Autodesk Inventor part; units mm, degrees
ref_plane "Work Plane1" through (0, 5, 0) normal (0, 1, 0) x (1, 0, 0)
ref_plane "Work Plane2" through (0, 80, 0) normal (0, 1, 0) x (1, 0, 0)
ref_plane "Work Plane3" through (-25, 0, 27) normal (0, 0, 1) x (1, 0, 0)
sketch "Sketch1" plane through (0, 0, 0) normal (0, 1, 0) x (-1, 0, 0)
  line L0 (27, 27) -> (-27, 27)
  line L1 (-27, 27) -> (-27, -27)
  line L2 (-27, -27) -> (27, -27)
  line L3 (27, -27) -> (27, 27)
  line L4 (27, 27) -> (-27, -27) construction
  line L5 (-27, 27) -> (27, -27) construction
  circle A0 centre (25, 25) radius 1
  circle A1 centre (25, -25) radius 1
  circle A2 centre (-25, -25) radius 1
  circle A3 centre (-25, 25) radius 1
  point P0 (0, 0)
  dimension "d0" = 54
  dimension "d1" = 54
  dimension "d2" = 2
  dimension "d3" = 2
  dimension "d4" = 2
  dimension "d5" = 2
extrude "Extrusion1" add sketch "Sketch1" along normal blind 5
fillet "Fillet1" radius 2 1 edges at (27, 2.5, -27)
fillet "Fillet2" radius 2 3 edges at (-27, 2.5, -27) (-27, 2.5, 27) (27, 2.5, 27)
ref_plane "Work Plane1" through (0, 5, 0) normal (0, 1, 0) x (1, 0, 0)
sketch "Sketch3" plane through (0, 5, 0) normal (0, 1, 0) x (1, 0, 0)
  circle A0 centre (0, 0) radius 25
  line L0 (-25, -27) -> (25, -27)
  line L1 (0, -27) -> (20, -27)
  line L2 (20, -27) -> (20, -15)
  line L3 (0, -27) -> (-20, -27)
  line L4 (-20, -27) -> (-20, -15)
  dimension "d11" = 50
  dimension "d12" = 20
  dimension "d13" = 20
extrude "Extrusion2" add sketch "Sketch3" along normal blind 75
ref_plane "Work Plane2" through (0, 80, 0) normal (0, 1, 0) x (1, 0, 0)
sketch "Sketch4" plane through (0, 80, 0) normal (0, 1, 0) x (1, 0, 0)
  circle A0 centre (0, 0) radius 20
  dimension "d17" = 40
extrude "Extrusion3" cut sketch "Sketch4" against normal blind 5
ref_plane "Work Plane3" through (-25, 0, 27) normal (0, 0, 1) x (1, 0, 0)
sketch "Sketch5" plane through (-25, 0, 27) normal (0, 0, 1) x (1, 0, 0)
  line L0 (25, 0) -> (25, 7.5)
  line L1 (5, 15) -> (45, 15)
  line L2 (45, 15) -> (45, 0)
  line L3 (45, 0) -> (5, 0)
  line L4 (5, 0) -> (5, 15)
  line L5 (5, 15) -> (45, 0) construction
  line L6 (45, 15) -> (5, 0) construction
  dimension "d21" = 7.5
  dimension "d22" = 40
  dimension "d23" = 15
extrude "Extrusion4" add sketch "Sketch5" along normal blind 5
ref_plane "Work Plane4" through (-25, 0, 32) normal (0, 0, 1) x (1, 0, 0)
sketch "Sketch6" plane through (-25, 0, 32) normal (0, 0, 1) x (1, 0, 0)
  line L0 (25, 7.5) -> (25, 8.92)
  circle A0 centre (25, 8.92) radius 0.5
  line L1 (25, 8.92) -> (27.3, 8.92)
  line L2 (27.3, 8.92) -> (29.6, 8.92)
  line L3 (25, 8.92) -> (22.7, 8.92)
  line L4 (22.7, 8.92) -> (20.4, 8.92)
  circle A1 centre (20.4, 8.92) radius 0.5
  circle A2 centre (27.3, 8.92) radius 0.5
  circle A3 centre (22.7, 8.92) radius 0.5
  circle A4 centre (29.6, 8.92) radius 0.5
  line L5 (25, 7.5) -> (25, 6.08)
  line L6 (26.15, 6.08) -> (25, 6.08)
  line L7 (23.85, 6.08) -> (25, 6.08)
  circle A5 centre (26.15, 6.08) radius 0.5
  circle A6 centre (23.85, 6.08) radius 0.5
  line L8 (23.85, 6.08) -> (21.55, 6.08)
  line L9 (26.15, 6.08) -> (28.45, 6.08)
  circle A7 centre (28.45, 6.08) radius 0.5
  circle A8 centre (21.55, 6.08) radius 0.5
  line L10 (18.3522, 10.2186) -> (31.6478, 10.2186)
  line L11 (30.8187, 4.7814) -> (19.1813, 4.7814)
  line L12 (31.6478, 10.2186) -> (30.8187, 4.7814)
  line L13 (18.3522, 10.2186) -> (19.1813, 4.7814)
  line L14 (25, 10.2186) -> (25, 11.0186)
  line L15 (25, 4.7814) -> (25, 3.9814)
  line L16 (25, 3.9814) -> (31.5285, 3.9814)
  line L17 (31.5285, 3.9814) -> (32.5973, 11.0186)
  line L18 (32.5973, 11.0186) -> (25, 11.0186)
  line L19 (25, 3.9814) -> (18.4715, 3.9814)
  line L20 (18.4715, 3.9814) -> (17.4027, 11.0186)
  line L21 (17.4027, 11.0186) -> (25, 11.0186)
  point P0 (25, 0)
  dimension "d30" = 1
  dimension "d33" = 1
  dimension "d34" = 1
  dimension "d35" = 1
  dimension "d36" = 1
  dimension "d38" = 1
  dimension "d39" = 1
  dimension "d40" = 1
  dimension "d41" = 1
  dimension "d44" = 0.8
extrude "Extrusion5" add sketch "Sketch6" along normal blind 10 contours A1 | A3 L4 L3 | L3 L4 A3 | A4 | A2 L2 L1 | L1 L2 A2 | A0 L3 L0 | L0 L1 A0 | A7 | A5 L9 L6 | L6 L9 A5 | A8 | A6 L8 L7 | L7 L8 A6 | L3 A0 L1 | L13 L11 L15 L19 L20 L21 L14 L10 | L14 L18 L17 L16 L15 L11 L12 L10
sketch "Sketch7" plane through (-25, 0, 32) normal (0, 0, 1) x (1, 0, 0)
  line L0 (5, 15) -> (5, 0)
  line L1 (5, 7.5) -> (10, 7.5)
  circle A0 centre (10, 7.5) radius 1.5
  line L2 (12.3579, 7.5) -> (11.1789, 5.458)
  line L3 (11.1789, 5.458) -> (8.8211, 5.458)
  line L4 (8.8211, 5.458) -> (7.6421, 7.5)
  line L5 (7.6421, 7.5) -> (8.8211, 9.542)
  line L6 (8.8211, 9.542) -> (11.1789, 9.542)
  line L7 (11.1789, 9.542) -> (12.3579, 7.5)
  line L8 (25, 0) -> (25, 2.1902)
  circle A1 centre (40, 7.5) radius 1.5
  line L9 (37.6421, 7.5) -> (38.8211, 5.458)
  line L10 (38.8211, 5.458) -> (41.1789, 5.458)
  line L11 (41.1789, 5.458) -> (42.3579, 7.5)
  line L12 (42.3579, 7.5) -> (41.1789, 9.542)
  line L13 (41.1789, 9.542) -> (38.8211, 9.542)
  line L14 (38.8211, 9.542) -> (37.6421, 7.5)
  dimension "d48" = 5
  dimension "d49" = 3
extrude "Extrusion6" add sketch "Sketch7" along normal blind 10
properties part number "sensor 1"
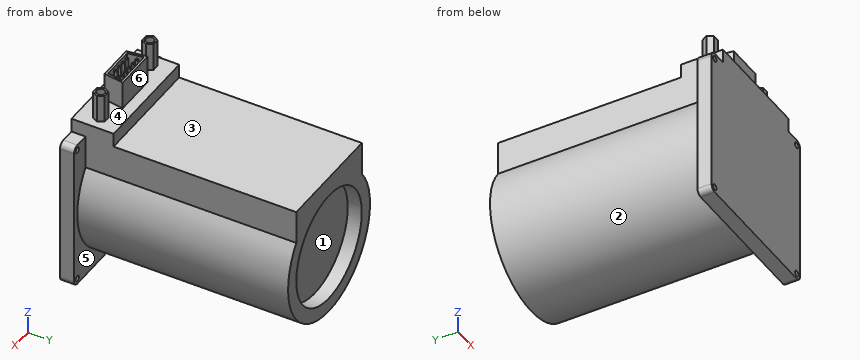
Read the model definition and answer for the solid it produces. Units are mm, in the model's axes. Face numbers are marked on the shaded views. A direction names the side the tool comes from. Round coordinates to 2 decimals unless told otherwise and drop trailing zeros. Loops run counter-clockwise (first coordinate to the right, second up) from the corner with the lowest first, then second, coordinate; pieces in that order, holes last.
Q1. Which of the six approach directions +Z, -Z, +X, -X, +Y, -Y give full straight-line access (tool end or side, diameter ignored) to the marked faces 4, 5 and 6?
Q2. Each of these flat-tipped pins is pushed along its axis until it touches: pin 1 (10 mm diameter, centred on y = 56, z = 0.5, fed in from -X); pin 2 (5 mm diameter, centred on x = -8, z = -3, fed in from +Y); pin 3 (3.5 mm diameter, centred on x = -15, y = 7.5, fed in from -Z); pin 4 (11 mm diameter, centred on x = 1, z = 35.5, fed in from -Y). Where does it stop, or does it pass through?
Q3. Section D-D on z = -6.5 is taken. Write down the section's boundary in (x, y).
Q4. Determine the mould class of the marked faces 1, 2 and 3 for opening direction X: released by +X, released by -X, zero draft, split by the parting line, or undercut.
Q5. Section C-C on z = 10 is taken. Write down the section's boundary in (x, y), and give its area (3 significant figures).
Q6. Section B-B on y = 13 is taken. Write down the section's boundary in (x, z).
Q7. Consider probe 1 along Z at (x, y) = (-25, 3.05); probe 2 along Y at (x, z) = (12, -13); probe 3 along X at (y, z) = (59.5, 23.5). Determine where each line is inside the solid, lowest interval first.
Q8. Section A-A on x = -15 is taken. Write down the section's boundary in (y, z), and give its area (3 significant figures).
Output:
1. face 4: +Z
1. face 5: +Y
1. face 6: +Z, +X, -X, +Y
2. pin 1: stops at x = -25
2. pin 2: stops at y = 75
2. pin 3: stops at z = -21.2
2. pin 4: stops at y = 0
3. outline: (-27, 0) - (27, 0) - (27, 5) - (24.14, 5) - (24.14, 80) - (18.91, 80) - (18.91, 75) - (-18.91, 75) - (-18.91, 80) - (-24.14, 80) - (-24.14, 5) - (-27, 5) - close
4. face 1: undercut
4. face 2: split by the parting line
4. face 3: zero draft
5. outline: (-27, 0) - (27, 0) - (27, 5) - (22.91, 5) - (22.91, 80) - (17.32, 80) - (17.32, 75) - (-17.32, 75) - (-17.32, 80) - (-22.91, 80) - (-22.91, 5) - (-27, 5) - close
5. area: 3,530 mm2
6. outline: (-20, 15) arc R25 ccw (long way) to (20, 15) - (20, 32) - (-20, 32) - close
7. probe 1: z = -27 to -26, -24 to 24, 26 to 27
7. probe 2: y = 0 to 75
7. probe 3: x = -20 to 20
8. outline: (0, -27) - (5, -27) - (5, -20) - (80, -20) - (80, -13.23) - (75, -13.23) - (75, 13.23) - (80, 13.23) - (80, 27) - (15, 27) - (15, 32) - (9.54, 32) - (9.54, 42) - (9, 42) - (9, 32) - (6, 32) - (6, 42) - (5.46, 42) - (5.46, 32) - (0, 32) - close
8. area: 3,750 mm2
